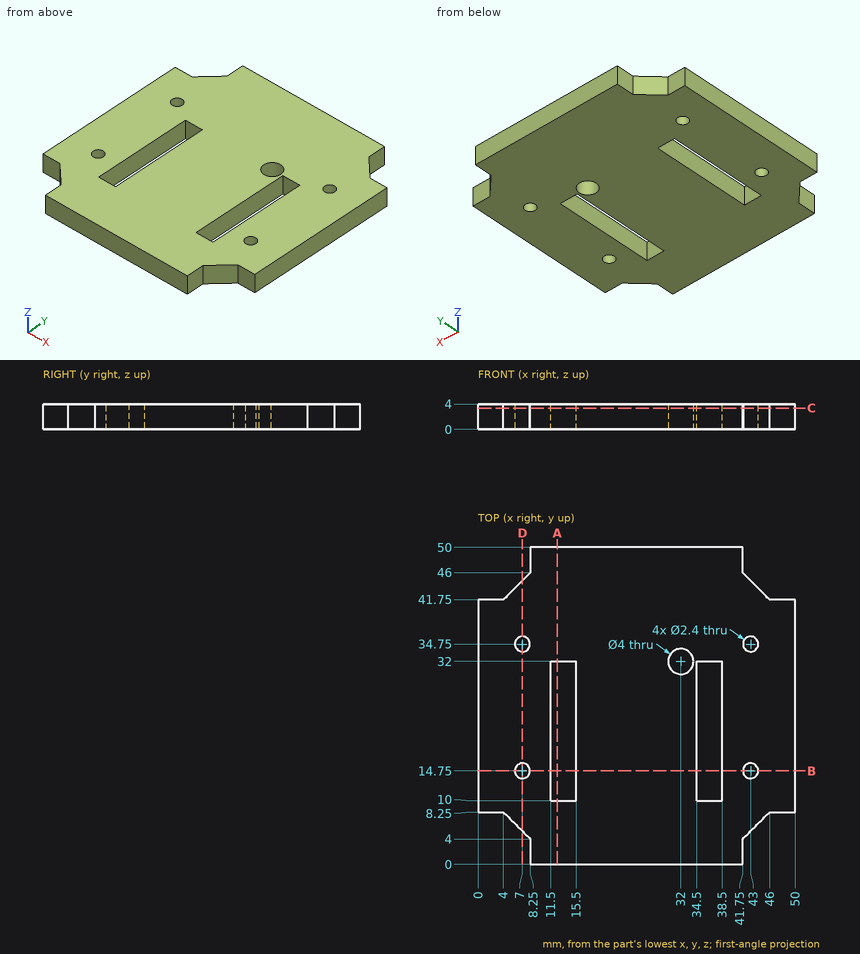
Input: dimensioned drawing with shaded views. Units: mm. Origin: part minimum x, y, z. Give positions to 0.01 mm unless a question says otherwise; leave off trailing zeros. Write each loop counter-clockwise with the first axis right and the second up, starting at its lowest first coordinate (ties: lowest second). Pieces come first, ordered by that corner, then holes.
1. Pin query (flat end, axial travel): P1, Ø2, axis at y = 48.5, z = 3, coming from the +X side; P2, Ø1.2, axis at x = 3, z = 2.5, coming from the +Y side; P3, Ø2, axis at y = 44.5, z = 1, coming from the -X side. Return the tip coordinate at first contact, or that it passes through.
2. Section query B-B, the plane y = 14.75. Return loops of the section in (x, z).
3. Section query A-A, the plane x = 12.5. Return loops of the section in (y, z), then the cut area to 3 significant figures.
4. Line query: probe 1 along X at (y, z) = (10.5, 1.35); probe 2 along Y at (x, z) = (36.5, 2.1); probe 3 along Y at (x, z) = (32, 1.25). Output: solid intervals per line, ascending.
5. Section query D-D, the plane x = 7. Return loops of the section in (y, z).
6. Section query C-C, the plane z = 3.35. Count the separate pieces of the cut face and the enclosed holes in it, then the cut area to 3 significant figures.
Computed:
1. P1: stops at x = 41.75
1. P2: stops at y = 41.75
1. P3: stops at x = 5.75
2. outline: (0, 0) - (5.8, 0) - (5.8, 4) - (0, 4) - close; (8.2, 0) - (11.5, 0) - (11.5, 4) - (8.2, 4) - close; (15.5, 0) - (34.5, 0) - (34.5, 4) - (15.5, 4) - close; (38.5, 0) - (41.8, 0) - (41.8, 4) - (38.5, 4) - close; (44.2, 0) - (50, 0) - (50, 4) - (44.2, 4) - close
3. outline: (0, 0) - (10, 0) - (10, 4) - (0, 4) - close; (32, 0) - (50, 0) - (50, 4) - (32, 4) - close
3. area: 112 mm2
4. probe 1: x = 0 to 11.5, 15.5 to 34.5, 38.5 to 50
4. probe 2: y = 0 to 10, 32 to 50
4. probe 3: y = 0 to 30, 34 to 50
5. outline: (5.25, 0) - (13.55, 0) - (13.55, 4) - (5.25, 4) - close; (15.95, 0) - (33.55, 0) - (33.55, 4) - (15.95, 4) - close; (35.95, 0) - (44.75, 0) - (44.75, 4) - (35.95, 4) - close
6. separate pieces: 1
6. enclosed holes: 7
6. area: 2,060 mm2
